```python
from build123d import *

# Parameters (mm, degrees)
BOSS_EXTRUDE1_DEPTH      = 32
BOSS_EXTRUDE1_DEPTH_BACK = 32
SKETCH2_W                = 96.2
SKETCH2_H                = 76.1
CUT_EXTRUDE1_DEPTH       = 32
CUT_EXTRUDE1_DEPTH_BACK  = 32
SKETCH3_R                = 4
CUT_EXTRUDE2_DEPTH       = 16.1
CUT_EXTRUDE2_DEPTH_BACK  = 16.1
SKETCH4_R                = 3.3
CUT_EXTRUDE3_DEPTH       = 4
CUT_EXTRUDE3_DEPTH_BACK  = 4
SKETCH5_R                = 3.3
CUT_EXTRUDE4_DEPTH       = 4
CUT_EXTRUDE4_DEPTH_BACK  = 4


with BuildPart() as part:
    # Sketch1 → Boss-Extrude1 (new body, two sides)
    with BuildSketch(Plane(origin=(0, 0, 0), x_dir=(0, 0, -1), z_dir=(1, 0, 0))) as boss_extrude1_sk:
        with BuildLine():
            Line((-8.05, 0), (8.05, 0))
            ThreePointArc((8.05, 0), (10.878427125, 1.171572875), (12.05, 4))
            Line((12.05, 4), (12.05, 40))
            Line((12.05, 40), (8.05, 40))
            Line((8.05, 40), (8.05, 5.6))
            ThreePointArc((8.05, 5.6), (7.58137085, 4.46862915), (6.45, 4))
            Line((6.45, 4), (-6.45, 4))
            ThreePointArc((-6.45, 4), (-7.58137085, 4.46862915), (-8.05, 5.6))
            Line((-8.05, 5.6), (-8.05, 40))
            Line((-8.05, 40), (-12.05, 40))
            Line((-12.05, 40), (-12.05, 4))
            ThreePointArc((-12.05, 4), (-10.878427125, 1.171572875), (-8.05, 0))
        make_face()
    extrude(amount=BOSS_EXTRUDE1_DEPTH)
    extrude(boss_extrude1_sk.sketch, amount=-BOSS_EXTRUDE1_DEPTH_BACK)

    # Sketch2 → Cut-Extrude1 (cut, two sides)
    with BuildSketch(Plane.XY) as cut_extrude1_sk:
        with Locations((0, 21.95)):
            Rectangle(SKETCH2_W, SKETCH2_H)
        with BuildLine():
            Line((0, 30), (0, 0))
            Line((0, 0), (32, 0))
            Line((32, 0), (32, 4))
            Line((32, 4), (19.19395406, 33.933345743))
            ThreePointArc((19.19395406, 33.933345743), (7.9924568, 39.796416197), (0, 30))
        make_face(mode=Mode.SUBTRACT)
    extrude(amount=CUT_EXTRUDE1_DEPTH, mode=Mode.SUBTRACT)
    extrude(cut_extrude1_sk.sketch, amount=-CUT_EXTRUDE1_DEPTH_BACK, mode=Mode.SUBTRACT)

    # Sketch3 → Cut-Extrude2 (cut, two sides)
    with BuildSketch(Plane.XY) as cut_extrude2_sk:
        with Locations((10, 30)):
            Circle(SKETCH3_R)
    extrude(amount=CUT_EXTRUDE2_DEPTH, mode=Mode.SUBTRACT)
    extrude(cut_extrude2_sk.sketch, amount=-CUT_EXTRUDE2_DEPTH_BACK, mode=Mode.SUBTRACT)

    # Sketch4 → Cut-Extrude3 (cut, two sides)
    with BuildSketch(Plane(origin=(0, 0, 0), x_dir=(1, 0, 0), z_dir=(0, 1, 0))) as cut_extrude3_sk:
        with Locations((6, 0)):
            Circle(SKETCH4_R)
    extrude(amount=CUT_EXTRUDE3_DEPTH, mode=Mode.SUBTRACT)
    extrude(cut_extrude3_sk.sketch, amount=-CUT_EXTRUDE3_DEPTH_BACK, mode=Mode.SUBTRACT)

    # Sketch5 → Cut-Extrude4 (cut, two sides)
    with BuildSketch(Plane(origin=(0, 0, 0), x_dir=(1, 0, 0), z_dir=(0, 1, 0))) as cut_extrude4_sk:
        with Locations((26, 0)):
            Circle(SKETCH5_R)
    extrude(amount=CUT_EXTRUDE4_DEPTH, mode=Mode.SUBTRACT)
    extrude(cut_extrude4_sk.sketch, amount=-CUT_EXTRUDE4_DEPTH_BACK, mode=Mode.SUBTRACT)


solid = part.part
```
Design review of the part built by this model. Coordinates are the model's own, in mm. A direction names the side the tool comes from. Round coordinates to 2 decimals unless told otherwise and drop trailing zeros. Write each loop counter-clockwise with the first axis right and the second up, starting at its lowest first coordinate (ties: lowest second). Pieces come first, ordered by that corner, then holes. Notation, with made-up numbers: (81.5, -22.5) -> (140.5, -22.5) arc R7 ccw to (140.5, -18.5) -> close; hole circle Ø10 at (51, -17.75). An arc over 180 degrees is marked (long way). Write item = value, one per line. Start each with the question number.
1) Mouldability with a two-part tool opening along Y and no side actions: class faces 1 (the face through (12, 19, -8.05)), 2 (the face through (9.479, 33.966, -10.022)), 3 (the face through (25.687, 18.757, -10.455)) as +Y half, -Y half, draft (parallel to the pull), parting line (faces both ways), or undercut.
2) Take a section at B-B, the plane x = 10. State the section outline as (y, z) points.
3) Tool access review of faces 4 (the face through (16, 4, 0)), 5 (the face through (0, 11.877, -8.202)): name each direction out of +Z, -Z, +X, -X, +Y, -Y from which nothing blocks a thin tool from reaching the whole face with its end or side.
4) Take a section at C-C, the plane y = 31. State the section outline as (x, z) points.
5) Clearance check with flat-ended pins moving along their axes: pin 1 (10 mm diameter, centred on y = 19, z = -8, fed in from +X); pin 2 (5 mm diameter, centred on y = 26, z = 8, fed in from +X); pin 3 (4 mm diameter, centred on x = 6, z = 0, fed in from -Y); pin 4 (4 mm diameter, centred on x = 9, z = 0.5, fed in from +Y). State where each tip first meets the part, or that it passes through.
6) Wall thickness on probe 1 along X at (y, z) = (2.15, 0); probe 2 along Z at (x, y) = (15.5, 29); probe 3 along Y at (x, z) = (10, -2): over which ranges is each line inside the solid? List them lowest first. Write a range as from..to.
7) Take a section at A-A, the plane z = 0. State the section outline as (x, y) points.
8) Take a section at D-D, the plane x = 25.5. State the section outline as (y, z) points.
Results list:
q1.face_1 = draft
q1.face_2 = undercut
q1.face_3 = +Y half
q2.outline = (0, -8.05) arc R4 ccw to (4, -12.05) -> (26, -12.05) -> (26, -8.05) -> (5.6, -8.05) arc R1.6 cw to (4, -6.45) -> (4, 6.45) arc R1.6 cw to (5.6, 8.05) -> (26, 8.05) -> (26, 12.05) -> (4, 12.05) arc R4 ccw to (0, 8.05) -> close; (34, -12.05) -> (40, -12.05) -> (40, -8.05) -> (34, -8.05) -> close; (34, 8.05) -> (40, 8.05) -> (40, 12.05) -> (34, 12.05) -> close
q3.face_4 = +X, -X, +Y
q3.face_5 = +Z, -Z, -X, +Y, -Y
q4.outline = (0.05, -12.05) -> (6.13, -12.05) -> (6.13, -8.05) -> (0.05, -8.05) -> close; (0.05, 8.05) -> (6.13, 8.05) -> (6.13, 12.05) -> (0.05, 12.05) -> close; (13.87, -12.05) -> (20.45, -12.05) -> (20.45, -8.05) -> (13.87, -8.05) -> close; (13.87, 8.05) -> (20.45, 8.05) -> (20.45, 12.05) -> (13.87, 12.05) -> close
q5.pin_1 = 27.72
q5.pin_2 = 23.66
q5.pin_3 = through
q5.pin_4 = 4
q6.probe_1 = 0..2.7, 9.3..22.7, 29.3..32
q6.probe_2 = -12.05..-8.05, 8.05..12.05
q6.probe_3 = 0..4
q7.outline = (0, 0) -> (2.7, 0) -> (2.7, 4) -> (0, 4) -> close; (9.3, 0) -> (22.7, 0) -> (22.7, 4) -> (9.3, 4) -> close; (29.3, 0) -> (32, 0) -> (32, 4) -> (29.3, 4) -> close
q8.outline = (0, -8.05) arc R4 ccw to (4, -12.05) -> (19.19, -12.05) -> (19.19, -8.05) -> (5.6, -8.05) arc R1.6 cw to (4, -6.45) -> (4, -3.26) -> (0, -3.26) -> close; (0, 3.26) -> (4, 3.26) -> (4, 6.45) arc R1.6 cw to (5.6, 8.05) -> (19.19, 8.05) -> (19.19, 12.05) -> (4, 12.05) arc R4 ccw to (0, 8.05) -> close
